Answer from the drawing. Dimensions are ordinates in mm from the lowest x, y and z of the part. A direction names the side the tool comes from. Coordinates: 2 decimals unless noted, no trailing zeros. Loops run counter-clockwise (first coordinate to the right, second up) from the corner with the lowest first, then second, coordinate; pieces in that order, holes last. Notation, with made-up numbers: (-39.75, 85) -> (9.25, 85) arc R12 ccw to (9.25, 98) -> close; hole circle Ø10 at (-38.5, 41). An arc over 180 degrees is marked (long way). Use a Markdown table: item, result.
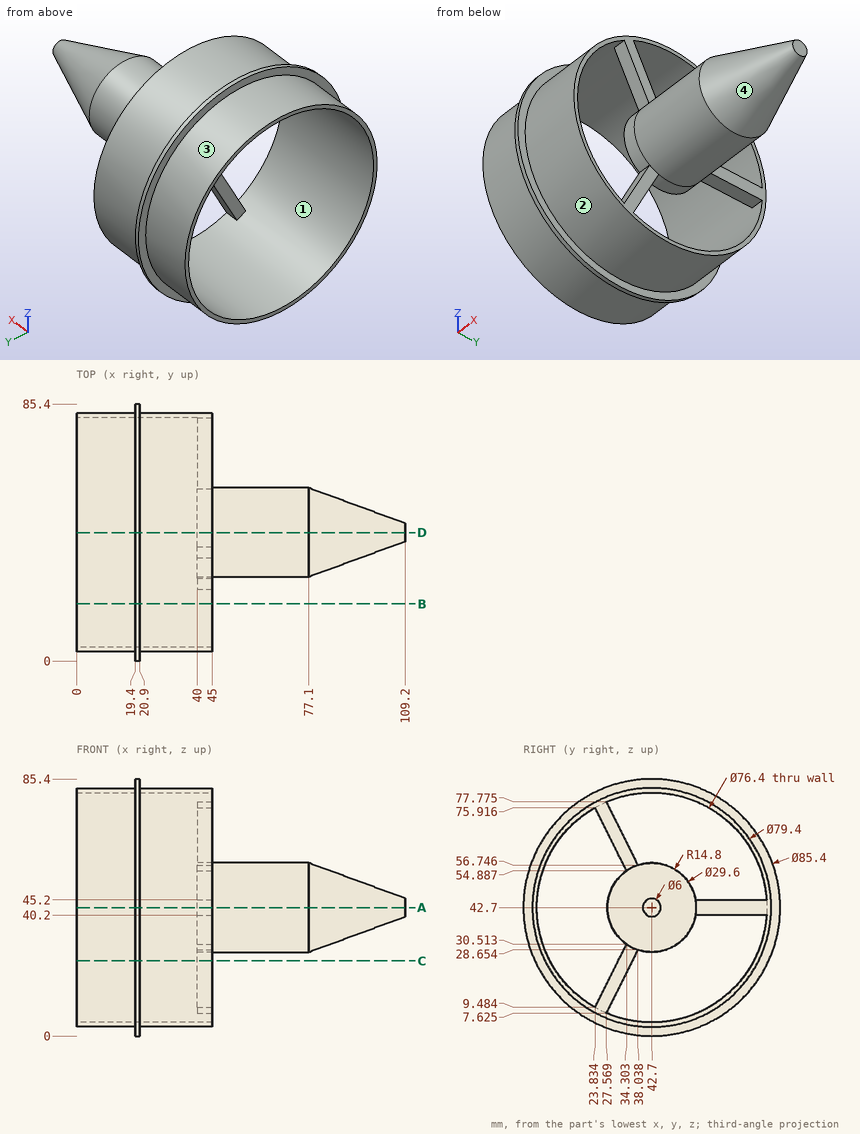
Q1. Determine the mould class of the marked faces 1 and 2 for opening direction Y: pulls with the +Y half, pulls with the -Y half, needs draft (parallel to the pull), parting line crosses it, or undercut.
Solved:
| item | result |
|---|---|
| face 1 | undercut |
| face 2 | parting line crosses it |
Q2. Section C-C on z = 25 is taken. Determine the outline of the cut face in (x, y) (1 decimal).
Solved:
| item | result |
|---|---|
| outline | (0, 7.2) -> (19.4, 7.2) -> (19.4, 3.8) -> (20.9, 3.8) -> (20.9, 7.2) -> (45, 7.2) -> (45, 8.8) -> (0, 8.8) -> close; (0, 76.6) -> (45, 76.6) -> (45, 78.2) -> (20.9, 78.2) -> (20.9, 81.6) -> (19.4, 81.6) -> (19.4, 78.2) -> (0, 78.2) -> close; (40, 31.6) -> (45, 31.6) -> (45, 36.2) -> (40, 36.2) -> close |
Q3. Consider line 1 (Z direction, x = 27, y = 42); line 2 (Y direction, x = 20, z = 42) (1 decimal). Determine where each line is inside the solid, lowest interval first. Write a range as [from, to].
Solved:
| item | result |
|---|---|
| line 1 | [3.01, 4.51], [80.89, 82.39] |
| line 2 | [0, 4.5], [80.9, 85.4] |
Q4. For the marked faces 3 and 4, determine the directions among +Z, -Z, +X, -X, +Y, -Y from which every point of the face is accessible in a straight line to the end or side of a thin tool.
Solved:
| item | result |
|---|---|
| face 3 | -X |
| face 4 | +X |
Q5. Section B-B on y = 19 is taken. Determine the outline of the cut face in (x, z), and give its area (3 significant figures).
Solved:
| item | result |
|---|---|
| outline | (0, 10.85) -> (19.4, 10.85) -> (19.4, 7.18) -> (20.9, 7.18) -> (20.9, 10.85) -> (45, 10.85) -> (45, 12.74) -> (0, 12.74) -> close; (0, 72.66) -> (45, 72.66) -> (45, 74.55) -> (20.9, 74.55) -> (20.9, 78.22) -> (19.4, 78.22) -> (19.4, 74.55) -> (0, 74.55) -> close |
| area | 181 mm² |
Q6. Section A-A on z = 42.7 is taken. Determine the outline of the cut face in (x, y), and give its area (3 significant figures).
Solved:
| item | result |
|---|---|
| outline | (0, 3) -> (19.4, 3) -> (19.4, 0) -> (20.9, 0) -> (20.9, 3) -> (45, 3) -> (45, 4.5) -> (0, 4.5) -> close; (0, 80.9) -> (40, 80.9) -> (40, 27.9) -> (77.1, 27.9) -> (109.2, 39.7) -> (109.2, 45.7) -> (77.1, 57.5) -> (45, 57.5) -> (45, 82.4) -> (20.9, 82.4) -> (20.9, 85.4) -> (19.4, 85.4) -> (19.4, 82.4) -> (0, 82.4) -> close |
| area | 1,930 mm² |
Q7. Section D-D on y = 42.7 is taken. State how many separate pieces and enclosed holes the cut face has, and give its area (3 significant figures).
Solved:
| item | result |
|---|---|
| separate pieces | 3 |
| enclosed holes | 0 |
| area | 1,810 mm² |
Q8. Given pin 1 Ø12 at (y, z) = (54, 51.5) entering from -X; pin 2 Ø10 at (x, y) = (98, 57.5) entering from +Z; pin 3 Ø3 at (y, z) = (63.5, 75.5) entering from -X; pin 4 Ø1.5 at (y, z) = (9.5, 66) entering from +X, each flat-ended and moving along its own axis, determine where each tip first touches the part or whether it passes through.
Solved:
| item | result |
|---|---|
| pin 1 | x = 40 |
| pin 2 | through |
| pin 3 | x = 0 |
| pin 4 | x = 20.9 |
